from build123d import *

# Parameters (mm, degrees)
ESBO_O1_R                       = 1.75
RESSALTO_EXTRUS_O1_DEPTH        = 16
ESBO_O3_R                       = 1.75
CORTE_EXTRUS_O2_DEPTH           = 30.470324057
CORTE_EXTRUS_O3_DEPTH           = 2
CORTE_EXTRUS_O3_TAPER           = 20
CORTE_EXTRUS_O3_OTHER_WAY_DEPTH = 6
CORTE_EXTRUS_O4_REACH           = 31.47
ESBO_O5_W                       = 29.879545061
ESBO_O5_H                       = 8
ESBO_O6_W                       = 11
ESBO_O6_H                       = 7
RESSALTO_EXTRUS_O2_DEPTH        = 3
ESBO_O7_W                       = 5.6
ESBO_O7_H                       = 2.5
CORTE_EXTRUS_O6_DEPTH           = 8
ESBO_O8_R                       = 1.65
CORTE_EXTRUS_O7_DEPTH           = 6
CHANFRO1_SIZE                   = 8


with BuildPart() as part:
    # Esboço1 → Ressalto-extrusão1 (new body)
    with BuildSketch(Plane.XY):
        with BuildLine():
            Line((17.5, 7.5), (6.986594306, 7.5))
            ThreePointArc((6.986594306, 7.5), (0, 10.25), (-6.986594306, 7.5))
            Line((-6.986594306, 7.5), (-17.5, 7.5))
            Line((-17.5, 7.5), (-17.5, -0.5))
            Line((-17.5, -0.5), (-7.232738071, -0.5))
            ThreePointArc((-7.232738071, -0.5), (-4.946589734, -5.300353762), (0, -7.25))
            Line((0, -7.25), (12.236067977, -7.25))
            Line((12.236067977, -7.25), (12.236067977, -4.75))
            Line((12.236067977, -4.75), (2.236067977, -4.75))
            ThreePointArc((2.236067977, -4.75), (-4.364690104, 2.917529829), (5.244044241, -0.25))
            Line((5.244044241, -0.25), (12.736067977, -0.25))
            Line((12.736067977, -0.25), (15.807189139, -0.25))
            Line((15.807189139, -0.25), (17.5, -0.25))
            Line((17.5, -0.25), (17.5, 7.5))
        make_face()
        with Locations((12.5, 3.5)):
            Circle(ESBO_O1_R, mode=Mode.SUBTRACT)
        with Locations(Location((-12.5, 3.5, 0), (0, 0, 180))):
            Circle(ESBO_O1_R, mode=Mode.SUBTRACT)
    extrude(amount=RESSALTO_EXTRUS_O1_DEPTH)

    # Esboço3 → Corte-extrusão2 (cut, through all)
    with BuildSketch(Plane.XZ.offset(7.25)):
        with Locations(Location((7.85, 12, 0), (0, 0, 240.437367967))):
            Circle(ESBO_O3_R)
    extrude(amount=-CORTE_EXTRUS_O2_DEPTH, mode=Mode.SUBTRACT)

    # Esboço4 → Corte-extrusão3 (cut)
    with BuildSketch(Plane(origin=(0, 7.5, 0), x_dir=(1, 0, 0), z_dir=(0, 1, 0))):
        Polygon((11.083161507, -12), (9.466580754, -9.2), (6.233419246, -9.2), (4.616838493, -12), (6.233419246, -14.8), (9.466580754, -14.8), align=None)
    extrude(amount=-CORTE_EXTRUS_O3_DEPTH, taper=CORTE_EXTRUS_O3_TAPER, mode=Mode.SUBTRACT)

    # Esboço4 → Corte-extrusão3 other way (cut)
    with BuildSketch(Plane(origin=(0, 7.5, 0), x_dir=(1, 0, 0), z_dir=(0, 1, 0))):
        Polygon((11.083161507, -12), (9.466580754, -9.2), (6.233419246, -9.2), (4.616838493, -12), (6.233419246, -14.8), (9.466580754, -14.8), align=None)
    extrude(amount=CORTE_EXTRUS_O3_OTHER_WAY_DEPTH, mode=Mode.SUBTRACT)

    # Corte-extrusão4: up to this face of the body (flat: up to its plane)
    corte_extrus_o4_end = Plane(part.part.faces().sort_by_distance((-12.366369035, -0.5, 8))[0])
    # Esboço5 → Corte-extrusão4 (cut, up to the picked face)
    with BuildSketch(Plane.XZ.offset(7.25), mode=Mode.PRIVATE) as corte_extrus_o4_sk1:
        with Locations((-2.703704553, 4)):
            Rectangle(ESBO_O5_W, ESBO_O5_H)
    corte_extrus_o4_tool1 = split(extrude(corte_extrus_o4_sk1.sketch, amount=-CORTE_EXTRUS_O4_REACH, mode=Mode.PRIVATE), bisect_by=corte_extrus_o4_end, keep=Keep.BOTH, mode=Mode.PRIVATE)
    add(corte_extrus_o4_tool1.solids().sort_by(Axis((-2.703705, -7.25, 4), (0, 1, 0)))[0], mode=Mode.SUBTRACT)

    # Esboço6 → Ressalto-extrusão2 (add)
    with BuildSketch(Plane.XZ.offset(0.25)):
        with Locations((12, 3.5)):
            Rectangle(ESBO_O6_W, ESBO_O6_H)
        with Locations((-12, 3.5)):
            Rectangle(ESBO_O6_W, ESBO_O6_H)
    extrude(amount=RESSALTO_EXTRUS_O2_DEPTH)

    # Esboço7 → Corte-extrusão6 (cut)
    with BuildSketch(Plane(origin=(0, 0, 0), x_dir=(-1, 0, 0), z_dir=(0, 0, -1))):
        with Locations((-12.5, 0.8)):
            Rectangle(ESBO_O7_W, ESBO_O7_H)
        with Locations((12.5, 0.8)):
            Rectangle(ESBO_O7_W, ESBO_O7_H)
    extrude(amount=-CORTE_EXTRUS_O6_DEPTH, mode=Mode.SUBTRACT)

    # Esboço8 → Corte-extrusão7 (cut)
    with BuildSketch(Plane.XZ.offset(3.25)):
        with Locations(Location((12.5, 4, 0), (0, 0, 270))):
            Circle(ESBO_O8_R)
        with Locations(Location((-12.5, 4, 0), (0, 0, 270))):
            Circle(ESBO_O8_R)
    extrude(amount=-CORTE_EXTRUS_O7_DEPTH, mode=Mode.SUBTRACT)

    # Chanfro1
    # the kernel refuses this chamfer: 8 mm, written as the material it takes off along each edge
    with BuildSketch(Plane(origin=(17.5, -20.823463904, 16), x_dir=(0.027495876610586487, 0, -0.9996219169112968), z_dir=(0, 1, 0))) as chanfro1_piece_1_section:
        Polygon((CHANFRO1_SIZE * 0.999621916911, CHANFRO1_SIZE * 0.0274958766106), (-CHANFRO1_SIZE * 0.0274958766106, CHANFRO1_SIZE * 0.999621916911), (0, 0), align=None)
    chanfro1_piece_1 = extrude(amount=48.896927807, mode=Mode.PRIVATE)
    chanfro1_piece_1 = split(chanfro1_piece_1, bisect_by=Plane(origin=(15.518542318, -4.75, 12.990728841), z_dir=(0, 1, 0)), keep=Keep.TOP, mode=Mode.PRIVATE)
    add(chanfro1_piece_1, mode=Mode.SUBTRACT)
    with BuildSketch(Plane(origin=(-17.5, 28.073463904, 16), x_dir=(0.9996219169112968, 0, 0.027495876610586494), z_dir=(0, -1, 0))) as chanfro1_piece_2:
        Polygon((CHANFRO1_SIZE * 0.999621916911, -CHANFRO1_SIZE * 0.0274958766106), (-CHANFRO1_SIZE * 0.0274958766106, -CHANFRO1_SIZE * 0.999621916911), (0, 0), align=None)
    extrude(amount=49.146927807, mode=Mode.SUBTRACT)


solid = part.part
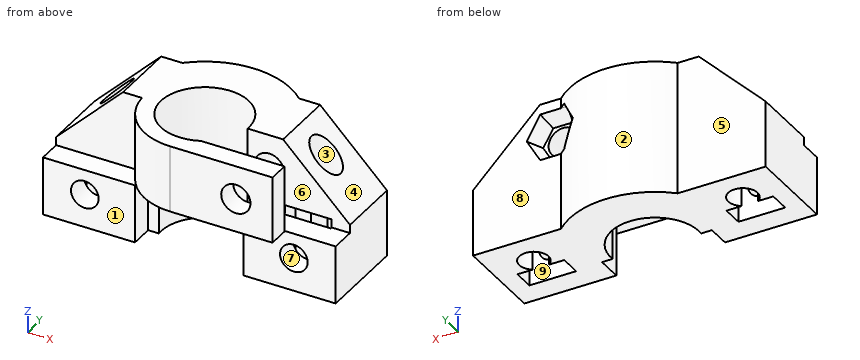
Geometry: final body of the model. Coordinates: model frame, mm. Face numbers are marked on the shaded views. A direction names the side the tool comes from. Round coordinates to 2 decimals unless told otherwise and drop trailing zeros. Loops run counter-clockwise (first coordinate to the right, second up) from the corner with the lowest first, then second, coordinate; pieces in that order, holes last. Notation, with made-up numbers: (-3, -22.5) - (50, -22.5) arc R14 ccw to (50, 2.5) - close; hole circle Ø2 at (39.5, 85.25). An arc over 180 degrees is marked (long way). Write each question's results on one line, items separated by ' | '. Start each with the question number.
1) Cut plane B-B on y = -2.75. Return loops of the section in (x, z), then the cut area to 3 significant figures.
2) Cut plane D-D on y = 3.5. Return loops of the section in (x, z).
3) Cut plane C-C on z = 6.5. Return loops of the section in (x, y), then the cut area to 3 significant figures.
4) First-contact query: P1, Ø4, axis at x = -6, z = 8, coming from the -Y side; P2, Ø0.8, axis at x = -13.5, y = -2.5, coming from the +Z side; P3, Ø2, axis at x = 10.5, z = 3, coming from the -Y side; P4, Ø8, axis at y = -5, z = 4.5, coming from the +X side. Flat tips, straight axial feed; report the tip coordinate or a pass-through.
5) Mould query, pull axis X, two halves, no side actions, for the marked faces 1, 2, 3 and 4. Classes: released by +X, released by -X, zero draft, split by the parting line, or undercut.
6) Access query for the marked faces 5, 6, 7, 8 and 9. Directions: +Z, -Z, +X, -X, +Y, -Y. A direction counts if a zero-diameter tool reaches every point of the face in a straight line with its end or side. Return the directions, or none.
7) Cut plane A-A on x = -12.5. Return loops of the section in (y, z).
8) Line query: probe 1 along X at (y, z) = (-1.6, 4); probe 2 along Y at (x, z) = (0, 12.25); probe 3 along Z at (x, y) = (7.85, -5.8). Output: solid intervals per line, ascending. Write a range as [from, to].
Verdict:
1) outline: (-17.5, 0) - (-6.5, 0) - (-6.5, 7) - (-17.5, 7) - close; (-6.71, 8) - (-4.47, 8) - (-4.47, 16) - (-6.71, 16) - close; (6.5, 0) - (17.5, 0) - (17.5, 7) - (6.5, 7) - close; hole circle Ø3.3 at (-12.5, 4); hole circle Ø3.3 at (12.5, 4) | area: 155 mm2
2) outline: (-17.5, 0) - (-14.25, 0) - (-14.25, 11.25) - (-17.5, 8) - close; (-10.75, 0) - (-3.91, 0) - (-3.91, 16) - (-9.5, 16) - (-10.75, 14.75) - close; (3.91, 0) - (10.75, 0) - (10.75, 14.75) - (9.5, 16) - (3.91, 16) - close; (14.25, 0) - (17.5, 0) - (17.5, 8) - (14.25, 11.25) - close; hole circle Ø3.5 at (7.85, 12)
3) outline: (-17.5, -3.25) - (-6.5, -3.25) - (-6.5, -0.5) - (-5.23, -0.5) arc R5.25 cw (long way) to (5.24, -0.25) - (6.5, -0.25) - (6.5, -3.25) - (17.5, -3.25) - (17.5, 7.5) - (6.99, 7.5) arc R10.25 ccw to (-6.99, 7.5) - (-17.5, 7.5) - close; hole (-15.3, -0.45) - (-9.7, -0.45) - (-9.7, 2.05) - (-11.52, 2.05) arc R1.75 ccw (long way) to (-13.48, 2.05) - (-15.3, 2.05) - close; hole (9.7, -0.45) - (15.3, -0.45) - (15.3, 2.05) - (13.48, 2.05) arc R1.75 ccw (long way) to (11.52, 2.05) - (9.7, 2.05) - close | area: 272 mm2
4) P1: stops at y = -6.05 | P2: stops at z = 7 | P3: stops at y = -3.25 | P4: stops at x = 17.5
5) face 1: zero draft | face 2: split by the parting line | face 3: undercut | face 4: released by +X
6) face 5: +Z, -Z, -X, +Y | face 6: +Z | face 7: -Y | face 8: +Z, -Z, +X, +Y | face 9: +Z, -Z
7) outline: (-3.25, 0) - (-0.45, 0) - (-0.45, 2.35) - (-3.25, 2.35) - close; (-3.25, 5.65) - (-0.45, 5.65) - (-0.45, 8) - (1.75, 8) - (1.75, 13) - (-0.5, 13) - (-0.5, 7) - (-3.25, 7) - close; (5.25, 0) - (7.5, 0) - (7.5, 13) - (5.25, 13) - close
8) probe 1: x = [-17.5, -14.15], [-10.85, -6.5], [6.5, 10.85], [14.15, 17.5] | probe 2: y = [-7.25, -5.25], [5.25, 10.25] | probe 3: z = [8, 10.25], [13.75, 16]
